Verification items for the finished model (mm, model axes). Face numbers are marked on the shaded views. Coordinates: 2 decimals unless noted, no trailing zeros. Order: outer loops, then holes, each group sorted by start corner. A loop starts at its lowest first (then second) coordinate and runs counter-clockwise, first axis right, second up. Notation, with made-up numbers: M 58.25,-40 L 112.25,-40 A31 cw 112.25,-4 Z; hole C 56,-37 d4. An arc over 180 degrees is marked long. Return JSON: item names as keys, results as strings. Group by question number.
Q1. Section check C-C, the plane z = 2.35. Enter the section's corners in (x, y) (3 decimals).
Q2. Mould release check, pull along X, two halves, no side actions. Record for the marked faces 1, 2 and 3: pulls with the +X half, pulls with the -X half, needs draft (parallel to the pull), parting line crosses it, or undercut.
Q3. Section check D-D, the plane x = -7. Enter the section's corners in (y, z), then the cut area to 3 significant figures.
Q4. Section check A-A, the plane y = 0. Enter the section's corners in (x, z).
Q5. Section check B-B, the plane x = 0. Enter the section's corners in (y, z).
Q6. Thickness scan on probe 1 along Y at (x, z) = (0, 0.2); probe 2 along Y at (x, z) = (-0.5, 1.85); probe 3 along X at (y, z) = (-0.5, 0.4). Record the ranges inside material, lowest first.
Q7. Go/stop test with a flat-tipped pin: pin 1 Ø1 at (y, z) = (8.5, 1.5) entering from -X. Record where the tip stops, or that it passes through.
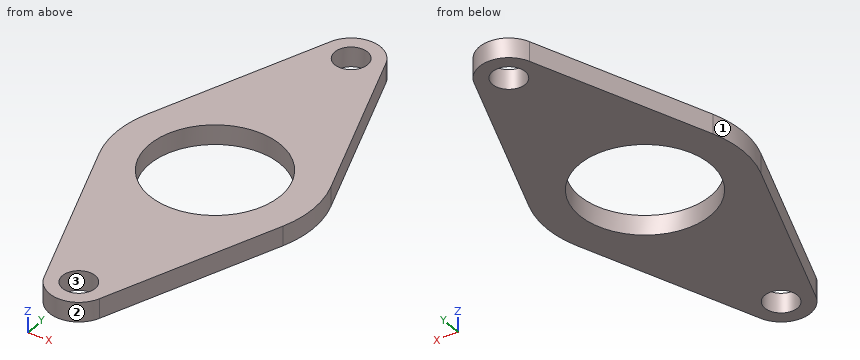
from build123d import *

# Parameters (mm, degrees)
SKETCH_1_R      = 2.5
SKETCH_1_R_2    = 10
EXTRUDE_1_DEPTH = 3


with BuildPart() as part:
    # 草图1 → 凸台-拉伸1 (new body)
    with BuildSketch(Plane.XY):
        with BuildLine():
            Line((-4.215373649, 31.575), (-14.051245496, 5.25))
            ThreePointArc((-14.051245496, 5.25), (-15, 0), (-14.051245496, -5.25))
            Line((-14.051245496, -5.25), (-4.215373649, -31.575))
            ThreePointArc((-4.215373649, -31.575), (0, -34.5), (4.215373649, -31.575))
            Line((4.215373649, -31.575), (14.051245496, -5.25))
            ThreePointArc((14.051245496, -5.25), (15, 0), (14.051245496, 5.25))
            Line((14.051245496, 5.25), (4.215373649, 31.575))
            ThreePointArc((4.215373649, 31.575), (0, 34.5), (-4.215373649, 31.575))
        make_face()
        with Locations((0, 30)):
            Circle(SKETCH_1_R, mode=Mode.SUBTRACT)
        with Locations((0, -30)):
            Circle(SKETCH_1_R, mode=Mode.SUBTRACT)
        Circle(SKETCH_1_R_2, mode=Mode.SUBTRACT)
    extrude(amount=EXTRUDE_1_DEPTH)


solid = part.part
Numbers:
{
 "1": {"outline": "M -14.051,-5.25 L -4.215,-31.575 A4.5 ccw 4.215,-31.575 L 14.051,-5.25 A15 ccw 14.051,5.25 L 4.215,31.575 A4.5 ccw -4.215,31.575 L -14.051,5.25 A15 ccw Z; hole C 0,0 d20; hole C 0,-30 d5; hole C 0,30 d5"},
 "2": {"face 1": "pulls with the -X half", "face 2": "parting line crosses it", "face 3": "undercut"},
 "3": {"outline": "M -24.12,0 L -7.14,0 L -7.14,3 L -24.12,3 Z; M 7.14,0 L 24.12,0 L 24.12,3 L 7.14,3 Z", "area": "102 mm2"},
 "4": {"outline": "M -15,0 L -10,0 L -10,3 L -15,3 Z; M 10,0 L 15,0 L 15,3 L 10,3 Z"},
 "5": {"outline": "M -34.5,0 L -32.5,0 L -32.5,3 L -34.5,3 Z; M -27.5,0 L -10,0 L -10,3 L -27.5,3 Z; M 10,0 L 27.5,0 L 27.5,3 L 10,3 Z; M 32.5,0 L 34.5,0 L 34.5,3 L 32.5,3 Z"},
 "6": {"probe 1": "y = -34.5 to -32.5, -27.5 to -10, 10 to 27.5, 32.5 to 34.5", "probe 2": "y = -34.47 to -32.45, -27.55 to -9.99, 9.99 to 27.55, 32.45 to 34.47", "probe 3": "x = -14.99 to -9.99, 9.99 to 14.99"},
 "7": {"pin 1": "stops at x = -13.02"}
}
